Check sheet for the modelled part. Datum: model origin and axes. Units: mm. A direction names the side the tool comes from. Give positions to 0.01 mm unless a question says otherwise; leave off trailing zeros. Write each loop counter-clockwise with the first axis right and the second up, starting at its lowest first coordinate (ties: lowest second). Pieces come first, ordered by that corner, then holes. Notation, with made-up numbers: (75.25, -8) -> (110.25, -8) arc R32 ccw to (110.25, 29) -> close; hole circle Ø7 at (42.25, 81.25). An arc over 180 degrees is marked (long way). Write each question's results on one line, items separated by ' | '. Start each with the question number.
```python
from build123d import *

# Parameters (mm, degrees)
F0_R      = 19.939
F1_DEPTH  = 19.05
F3_R      = 6.3754
F4_DEPTH  = 12.7
F5_R      = 3.8354
F6_DEPTH  = 6.351
F8_DEPTH  = 38.1
F10_DEPTH = 38.1


with BuildPart() as f1:
    # F0 (on Top) → F1 (new body)
    with BuildSketch(Plane.XY):
        Circle(F0_R)
    extrude(amount=F1_DEPTH)

    # F3 (on face) → F4 (cut)
    with BuildSketch(Plane(origin=(0, 0, 0), x_dir=(1, 0, 0), z_dir=(0, 0, -1))):
        with Locations((-9.519071, 0)):
            Circle(F3_R)
        with Locations((0, 9.519071)):
            Circle(F3_R)
        with Locations((9.519071, 0)):
            Circle(F3_R)
        with Locations((0, -9.519071)):
            Circle(F3_R)
    extrude(amount=-F4_DEPTH, mode=Mode.SUBTRACT)

    # F5 (on face) → F6 (cut, through all)
    with BuildSketch(Plane(origin=(0, 0, 12.7), x_dir=(1, 0, 0), z_dir=(0, 0, -1))):
        with Locations((0, 9.519071)):
            Circle(F5_R)
        with Locations((-9.519071, 0)):
            Circle(F5_R)
        with Locations((0, -9.519071)):
            Circle(F5_R)
        with Locations((9.519071, 0)):
            Circle(F5_R)
    extrude(amount=-F6_DEPTH, mode=Mode.SUBTRACT)

    # F7 (on Front) → F8 (cut, symmetric)
    with BuildSketch(Plane.XZ):
        Polygon((-8.64362, 23.88362), (0, 15.24), (8.64362, 23.88362), align=None)
    extrude(amount=F8_DEPTH, both=True, mode=Mode.SUBTRACT)

    # F9 (on Right) → F10 (cut, symmetric)
    with BuildSketch(Plane.YZ):
        Polygon((-11.610578, 26.850578), (0, 15.24), (11.610578, 26.850578), align=None)
    extrude(amount=F10_DEPTH, both=True, mode=Mode.SUBTRACT)


solid = f1.part
```
Item 1: Section check B-B on y = -1.5. Record the boundary of the cut face in (x, z).
Item 2: Set-up check for faces 1 (the cylindrical face through (-1.382, 15.743, 6.261)), 2 (the cylindrical face through (13.06, 1.47, 15.12)), 3 (the flat face through (-15.99, -1.93, 17.17)), 4 (the flat face through (-1.93, 15.99, 17.17)): record each of +Z, -Z, +X, -X, +Y, -Y from which the full face is reachable in a straight line by a thin tool's end or side.
Item 3: Section check C-C on z = 16. Record the boundary of the cut face in (x, y).
Item 4: Depth check by flat-ended pin: pin 1 Ø9 at (x, y) = (-9.52, 0) entering from -Z; pin 2 Ø10 at (y, z) = (-8.5, 8) entering from -X; pin 3 Ø10 at (x, z) = (-10, 15.5) entering from +Y. Enter the tip coordinate at first touch or a pass-through.
Item 5: Section check A-A on x = 2. Record the boundary of the cut face in (y, z), then the cut area to 3 significant figures.
Item 6: Section check D-D on y = -11. Record the boundary of the cut face in (x, z).
Item 7: Mould release check, pull along Y, two halves, no side actions. Record for faces 5 (the cylindrical face through (18.419, -7.637, 9.392)), 6 (the flat face through (10, 10, 19.05)), 7 (the flat face through (4.6, -1.93, 17.17)): pulls with the +Y half, pulls with the -Y half, needs draft (parallel to the pull), parting line crosses it, or undercut.
Item 8: Thickness scan on probe 1 along X at (y, z) = (0, 2.75); probe 2 along X at (y, z) = (-1, 4.25); probe 3 along Y at (x, z) = (5.5, 9.5). Record the ranges inside material, lowest first. Write a range as from..to.
Check sheet entries:
1) outline: (-19.88, 0) -> (-15.72, 0) -> (-15.72, 12.7) -> (-13.05, 12.7) -> (-13.05, 16.74) -> (-19.88, 16.74) -> close; (-5.99, 12.7) -> (-3.32, 12.7) -> (-3.32, 0) -> (3.32, 0) -> (3.32, 12.7) -> (5.99, 12.7) -> (5.99, 16.74) -> (1.5, 16.74) -> (0, 15.24) -> (-1.5, 16.74) -> (-5.99, 16.74) -> close; (13.05, 12.7) -> (15.72, 12.7) -> (15.72, 0) -> (19.88, 0) -> (19.88, 16.74) -> (13.05, 16.74) -> close
2) face 1: -Z | face 2: +Z, -Z | face 3: +Z, +X, -X | face 4: +Z, +Y, -Y
3) outline: (-19.92, -0.76) arc R19.94 ccw to (-0.76, -19.92) -> (-0.76, -13.28) arc R3.84 cw to (-0.76, -5.76) -> (-0.76, -0.76) -> (-5.76, -0.76) arc R3.84 cw to (-13.28, -0.76) -> close; (-19.92, 0.76) -> (-13.28, 0.76) arc R3.84 cw to (-5.76, 0.76) -> (-0.76, 0.76) -> (-0.76, 5.76) arc R3.84 cw to (-0.76, 13.28) -> (-0.76, 19.92) arc R19.94 ccw to start; (0.76, -19.92) arc R19.94 ccw to (19.92, -0.76) -> (13.28, -0.76) arc R3.84 cw to (5.76, -0.76) -> (0.76, -0.76) -> (0.76, -5.76) arc R3.84 cw to (0.76, -13.28) -> close; (0.76, 0.76) -> (5.76, 0.76) arc R3.84 cw to (13.28, 0.76) -> (19.92, 0.76) arc R19.94 ccw to (0.76, 19.92) -> (0.76, 13.28) arc R3.84 cw to (0.76, 5.76) -> close
4) pin 1: stops at z = 12.7 | pin 2: stops at x = -19.63 | pin 3: stops at y = 19.3
5) outline: (-19.84, 0) -> (-15.57, 0) -> (-15.57, 12.7) -> (-12.79, 12.7) -> (-12.79, 17.24) -> (-19.84, 17.24) -> close; (-6.25, 12.7) -> (-3.47, 12.7) -> (-3.47, 0) -> (3.47, 0) -> (3.47, 12.7) -> (6.25, 12.7) -> (6.25, 17.24) -> (2, 17.24) -> (0, 15.24) -> (-2, 17.24) -> (-6.25, 17.24) -> close; (12.79, 12.7) -> (15.57, 12.7) -> (15.57, 0) -> (19.84, 0) -> (19.84, 17.24) -> (12.79, 17.24) -> close | area: 313 mm^2
6) outline: (-16.63, 0) -> (-6.2, 0) -> (-6.2, 12.7) -> (-3.54, 12.7) -> (-3.54, 18.78) -> (-3.81, 19.05) -> (-16.63, 19.05) -> close; (3.54, 12.7) -> (6.2, 12.7) -> (6.2, 0) -> (16.63, 0) -> (16.63, 19.05) -> (3.81, 19.05) -> (3.54, 18.78) -> close
7) face 5: parting line crosses it | face 6: needs draft | face 7: undercut
8) probe 1: x = -19.94..-15.89, -3.14..3.14, 15.89..19.94 | probe 2: x = -19.91..-15.82, -3.22..3.22, 15.82..19.91 | probe 3: y = -19.17..-12.74, -6.29..-4.95, 4.95..6.29, 12.74..19.17
